Autodesk Inventor part; units mm, degrees
ref_plane "YZ Plane" through (0, 0, 0) normal (1, 0, 0) x (0, 1, 0)
ref_plane "XZ Plane" through (0, 0, 0) normal (0, 1, 0) x (-1, 0, 0)
ref_plane "XY Plane" through (0, 0, 0) normal (0, 0, 1) x (1, 0, 0)
sketch "Sketch1" plane through (0, 0, 0) normal (0, 1, 0) x (-1, 0, 0)
  circle A0 centre (0, 0) radius 1.65
  circle A1 centre (0, -12) radius 1.65
  line L0 (-5, 5.5) -> (5, 5.5)
  line L1 (5, 5.5) -> (5, -17.5)
  line L2 (5, -17.5) -> (-5, -17.5)
  line L3 (-5, -17.5) -> (-5, 5.5)
  dimension "d0" = 3.3
  dimension "d1" = 3.3
  dimension "d2" = 12
  dimension "d3" = 0
  dimension "d4" = 10
  dimension "d5" = 5
  dimension "d6" = 5.5
  dimension "d7" = 5.5
extrude "Extrusion1" add sketch "Sketch1" along normal blind 5
fillet "Fillet1" radius 2 4 edges at (5, 2.5, 5.5) (-5, 2.5, 5.5) (5, 2.5, -17.5) (-5, 2.5, -17.5)
properties part number "BeltClip"
Verification items for the finished model (mm, model axes). Coordinates: 2 decimals unless noted, no trailing zeros. Order: outer loops, then holes, each group sorted by start corner. A loop starts at its lowest first (then second) coordinate and runs counter-clockwise, first axis right, second up. Notation, with made-up numbers: M -14,-23.5 L 44,-23.5 A18 ccw 44,-2.5 Z; hole C 85,-37.75 d9. An arc over 180 degrees is marked long. Return JSON: item names as keys, results as strings.
1) Cross-section at B-B, the plane z = 0. Record the boundary of the cut face in (x, y).
Answer list:
{"outline": "M -5,0 L -1.65,0 L -1.65,5 L -5,5 Z; M 1.65,0 L 5,0 L 5,5 L 1.65,5 Z"}
2) Gauge pin test, flat end, axial feed: pin 1 (6 mm diameter, centred on x = 4, z = -4, fed in from -Y). Record the tip position at first contact, or that the pin passes through.
Answer list:
{"pin 1": "y = 0"}
3) Release check for a two-part mould opening along Z. For faces 1 (the flat face through (5, 2, -6)), 2 (the cylindrical face through (4.43, 2.54, -16.9)), 3 (the cylindrical face through (0.4, 2.5, -10.4)), 4 (the cylindrical face through (-4.43, 2.54, 4.9)) record: +Z half, -Z half, draft (parallel to the pull), parting line (faces both ways), or undercut.
Answer list:
{"face 1": "draft", "face 2": "-Z half", "face 3": "undercut", "face 4": "+Z half"}
4) Cross-section at C-C, the plane y = 4.4. Record the boundary of the cut face in (x, z), and give its area (3 significant figures).
Answer list:
{"outline": "M -5,-15.5 A2 ccw -3,-17.5 L 3,-17.5 A2 ccw 5,-15.5 L 5,3.5 A2 ccw 3,5.5 L -3,5.5 A2 ccw -5,3.5 Z; hole C 0,-12 d3.3; hole C 0,0 d3.3", "area": "209 mm2"}
5) Cross-section at D-D, the plane x = 1. Record the boundary of the cut face in (y, z).
Answer list:
{"outline": "M 0,-17.5 L 5,-17.5 L 5,-13.31 L 0,-13.31 Z; M 0,-10.69 L 5,-10.69 L 5,-1.31 L 0,-1.31 Z; M 0,1.31 L 5,1.31 L 5,5.5 L 0,5.5 Z"}
6) Thickness scan on L1, parallel to Z at x = 0, y = 2.9; L2, parallel to Z at x = -1.5, y = 3.5; L3, parallel to X at y = 4.3, z = -12.5. Record the ranges inside material, lowest first. Write a range as [from, to].
Answer list:
{"L1": "[-17.5, -13.65], [-10.35, -1.65], [1.65, 5.5]", "L2": "[-17.5, -12.69], [-11.31, -0.69], [0.69, 5.5]", "L3": "[-5, -1.57], [1.57, 5]"}
7) Cross-section at A-A, the plane x = 0. Record the boundary of the cut face in (y, z).
Answer list:
{"outline": "M 0,-17.5 L 5,-17.5 L 5,-13.65 L 0,-13.65 Z; M 0,-10.35 L 5,-10.35 L 5,-1.65 L 0,-1.65 Z; M 0,1.65 L 5,1.65 L 5,5.5 L 0,5.5 Z"}
